Design review of the part built by this model. Coordinates are the model's own, in mm. Face numbers are marked on the shaded views. Coordinates: 2 decimals unless noted, no trailing zeros. Loops run counter-clockwise (first coordinate to the right, second up) from the corner with the lowest first, then second, coordinate; pieces in that order, holes last. Notation, with made-up numbers: (29.25, -12) - (85.25, -12) arc R34 ccw to (85.25, 21) - close; hole circle Ø8 at (89, 67). An arc over 180 degrees is marked (long way). One line per question, with ' | ' between items.
from build123d import *

# Parameters (mm, degrees)
F3_R          = 1
F4_SIZE       = 1
F5_W          = 50
F5_H          = 14
F6_DEPTH      = 0.5
F6_DEPTH_BACK = 0.5
F7_COUNT      = 3


with BuildPart() as f2:
    # F1 (on Front) → F2 (revolve)
    with BuildSketch(Plane.XZ):
        Polygon((0, 2), (0, 0), (14, 0), (14, 12.5), (12, 12.5), (12, 8), (12, 2), align=None)
        with BuildLine():
            Line((12, 8), (12, 12.5))
            ThreePointArc((12, 12.5), (11.4651427749, 10.25), (12, 8))
        make_face()
    revolve(axis=Axis((0, 0, 9.526854381), (0, 0, 1)))

    # F3
    f3_edges = [f2.edges().sort_by_distance(p)[0] for p in [
        (-12, 0, 12.5),
    ]]
    fillet(f3_edges, radius=F3_R)

    # F4
    f4_edges = [f2.edges().sort_by_distance(p)[0] for p in [
        (-14, 0, 0),
    ]]
    chamfer(f4_edges, length=F4_SIZE)


with BuildPart() as f6:
    # F5 (on Front) → F6 (new body, two sides)
    with BuildSketch(Plane.XZ) as f6_sk:
        with Locations((0, 11)):
            Rectangle(F5_W, F5_H)
    extrude(amount=F6_DEPTH)
    extrude(f6_sk.sketch, amount=-F6_DEPTH_BACK)


with BuildPart() as f7_1:
    # F7: instance of F6
    add(f6.part.rotate(Axis((0, 0, 20.1674159616), (0, 0, 1)), 1 * 360 / F7_COUNT))


with BuildPart() as f7_2:
    # F7: instance of F6
    add(f6.part.rotate(Axis((0, 0, 20.1674159616), (0, 0, 1)), 2 * 360 / F7_COUNT))


with BuildPart() as f2_1:
    add(f2.part)

    # F8: cut F7_1, F6, F7_2
    add(f7_1.part, mode=Mode.SUBTRACT)
    add(f6.part, mode=Mode.SUBTRACT)
    add(f7_2.part, mode=Mode.SUBTRACT)


solid = f2_1.part
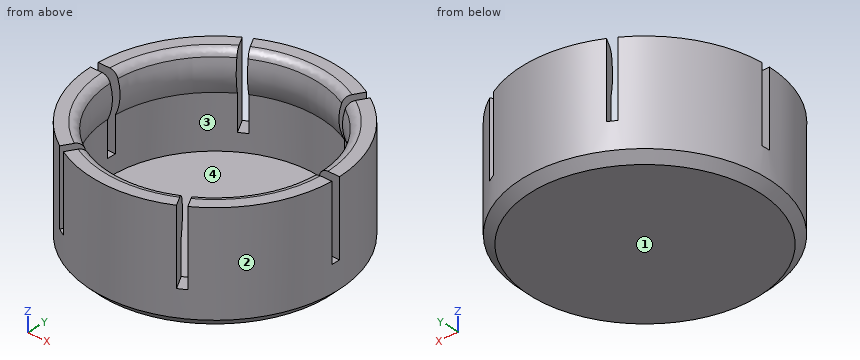
Q1. Take a section at B-B (y = 0). Give the boundary of the cut face in (x, z), plus the area to 3 significant figures.
Returned:
outline: (-14, 1) - (-13, 0) - (13, 0) - (14, 1) - (14, 4) - (12, 4) - (12, 2) - (-12, 2) - (-12, 4) - (-14, 4) - close | area: 63.0 mm²
Q2. Take a section at C-C (z = 4.5). Give the boundary of the cut face in (x, y).
Returned:
outline: (-13.99, -0.5) arc R14 ccw to (-7.43, -11.87) - (-6.43, -10.13) arc R12 cw to (-11.99, -0.5) - close; (-13.99, 0.5) - (-11.99, 0.5) arc R12 cw to (-6.43, 10.13) - (-7.43, 11.87) arc R14 ccw to start; (-6.56, -12.37) arc R14 ccw to (6.56, -12.37) - (5.56, -10.63) arc R12 cw to (-5.56, -10.63) - close; (-6.56, 12.37) - (-5.56, 10.63) arc R12 cw to (5.56, 10.63) - (6.56, 12.37) arc R14 ccw to start; (6.43, -10.13) - (7.43, -11.87) arc R14 ccw to (13.99, -0.5) - (11.99, -0.5) arc R12 cw to start; (6.43, 10.13) arc R12 cw to (11.99, 0.5) - (13.99, 0.5) arc R14 ccw to (7.43, 11.87) - close
Q3. To check wall thickness, follow line 1 along Y through (x, z) = (0, 5); line 2 along Z through (x, y) = (-0.75, 1.25). State the ranges of each line that lie inside material, in increasing order.
Returned:
line 1: y = -14 to -12, 12 to 14 | line 2: z = 0 to 2
Q4. For pin 1 (1.5 mm diameter, centred on y = -2, z = 2, fed in from +X); pin 2 (3 mm diameter, centred on y = 5.5, z = 9, fed in from +X); pin 3 (6 mm diameter, centred on x = -8, y = -5, fed in from +Z), all flat-tipped, find the tip position at first contact; note any pin that passes through.
Returned:
pin 1: stops at x = 13.94 | pin 2: stops at x = 13.42 | pin 3: stops at z = 12.47
Q5. Draft analysis for pull direction X (two halves, no side actions). For the marked faces 1, 2, 3 and 4, state which applies: +X half, -X half, draft (parallel to the pull), parting line (faces both ways), or undercut.
Returned:
face 1: draft | face 2: parting line | face 3: undercut | face 4: undercut
Q6. Take a section at A-A (z = 10.5). Give the boundary of the cut face in (x, y).
Returned:
outline: (-13.99, -0.5) arc R14 ccw to (-7.43, -11.87) - (-6.16, -9.68) arc R11.47 cw to (-11.46, -0.5) - close; (-13.99, 0.5) - (-11.46, 0.5) arc R11.47 cw to (-6.16, 9.68) - (-7.43, 11.87) arc R14 ccw to start; (-6.56, -12.37) arc R14 ccw to (6.56, -12.37) - (5.3, -10.18) arc R11.47 cw to (-5.3, -10.18) - close; (-6.56, 12.37) - (-5.3, 10.18) arc R11.47 cw to (5.3, 10.18) - (6.56, 12.37) arc R14 ccw to start; (6.16, -9.68) - (7.43, -11.87) arc R14 ccw to (13.99, -0.5) - (11.46, -0.5) arc R11.47 cw to start; (6.16, 9.68) arc R11.47 cw to (11.46, 0.5) - (13.99, 0.5) arc R14 ccw to (7.43, 11.87) - close
